Model file for the job. Use its own axes, mm. A direction names the side the tool comes from. Give positions to 0.01 mm unless a question says otherwise; leave off trailing zeros. Loops run counter-clockwise (first coordinate to the right, second up) from the corner with the lowest first, then second, coordinate; pieces in that order, holes last. Notation, with made-up numbers: M -26.5,29.5 L 7.5,29.5 A33 cw 7.5,61.5 Z; hole C 53.5,32 d2. An arc over 180 degrees is marked long. Answer in a Markdown table with one row per item.
```python
from build123d import *

# Parameters (mm, degrees)
EXTRUDE1_DEPTH      = 5.08
EXTRUDE1_DEPTH_BACK = 5.08
SKETCH3_R           = 9.525
SKETCH4_R           = 2.5796875
CUT_EXTRUDE1_DEPTH  = 37.55526843
FILLET1_R           = 2.54
FILLET2_R           = 2.54
CHAMFER1_SIZE       = 0.127
FILLET3_R           = 0.254
CHAMFER2_SIZE       = 0.127


with BuildPart() as part:
    # Sketch3 → Extrude1 (new, two sides: drawn at the far end of the back side and taken through both)
    with BuildSketch(Plane.XY.offset(-EXTRUDE1_DEPTH_BACK)):
        with BuildLine():
            Line((14.2875, 0), (14.2875, -7.9375))
            Line((14.2875, -7.9375), (28.575, -7.9375))
            Line((28.575, -7.9375), (28.575, -14.2875))
            Line((28.575, -14.2875), (-28.575, -14.2875))
            Line((-28.575, -14.2875), (-28.575, -7.9375))
            Line((-28.575, -7.9375), (-14.2875, -7.9375))
            Line((-14.2875, -7.9375), (-14.2875, 0))
            ThreePointArc((-14.2875, 0), (0, 14.2875), (14.2875, 0))
        make_face()
        Circle(SKETCH3_R, mode=Mode.SUBTRACT)
    extrude(amount=EXTRUDE1_DEPTH + EXTRUDE1_DEPTH_BACK)

    # Sketch4 → Cut-Extrude1 (cut, through all)
    with BuildSketch(Plane(origin=(0, -7.9375, 0), x_dir=(1, 0, 0), z_dir=(0, 1, 0))):
        with Locations(Location((-22.225, 0, 0), (0, 0, 270))):
            Circle(SKETCH4_R)
        with Locations(Location((22.225, 0, 0), (0, 0, 270))):
            Circle(SKETCH4_R)
        Polygon((-28.575, 5.08), (-28.575, 2.54), (-26.035, 5.08), align=None)
        Polygon((26.035, 5.08), (28.575, 5.08), (28.575, 2.54), align=None)
        Polygon((28.575, -5.08), (28.575, -2.54), (26.035, -5.08), align=None)
        Polygon((-26.035, -5.08), (-28.575, -5.08), (-28.575, -2.54), align=None)
    extrude(amount=-CUT_EXTRUDE1_DEPTH, mode=Mode.SUBTRACT)

    # Fillet1
    fillet1_edges = [part.edges().sort_by_distance(p)[0] for p in [
        (0, 14.2875, -5.08),
        (14.2875, -3.96875, -5.08),
        (14.2875, -3.96875, 5.08),
        (-14.2875, -3.96875, -5.08),
        (0, 14.2875, 5.08),
        (-14.2875, -3.96875, 5.08),
    ]]
    fillet(fillet1_edges, radius=FILLET1_R)

    # Fillet2
    # the kernel refuses this fillet: 2.54 mm, written as the material it adds along each edge
    with BuildSketch(Plane(origin=(-14.2875, -7.9375, -2.54), x_dir=(0, 1, 0), z_dir=(0, 0, 1)), Plane(origin=(14.2875, -7.9375, 2.54), x_dir=(0, 1, 0), z_dir=(0, 0, -1))) as fillet2_piece_1:
        with BuildLine():
            CenterArc((FILLET2_R, FILLET2_R), FILLET2_R, 180, 90)
            Line((0, FILLET2_R), (0, 0))
            Line((0, 0), (FILLET2_R, 0))
        make_face()
    extrude(amount=5.08)
    with BuildSketch(Plane(origin=(11.7475, -7.9375, -2.54), x_dir=(-0.5976672776328281, 0, 0.8017442392976479), z_dir=(0.8017442392976479, 0, 0.5976672776328281))) as fillet2_piece_2_section:
        with BuildLine():
            CenterArc((2.54 + FILLET2_R, -FILLET2_R), FILLET2_R, 90, 90)
            Line((2.54 + FILLET2_R, 0), (2.54, 0))
            Line((2.54, 0), (2.54, -FILLET2_R))
        make_face()
    fillet2_piece_2 = revolve(axis=Axis((11.7475, -7.9375, -2.54), (0, -1, 0)), revolution_arc=233.296989237, mode=Mode.PRIVATE)
    fillet2_piece_2 = split(fillet2_piece_2, bisect_by=Plane(origin=(13.652344814, -7.145963779, -5.08), z_dir=(0, 0, 1)), keep=Keep.TOP, mode=Mode.PRIVATE)
    add(fillet2_piece_2)
    with BuildSketch(Plane(origin=(-11.7475, -7.9375, -2.54), x_dir=(0.5976672776328252, 0, 0.8017442392976498), z_dir=(-0.8017442392976498, 0, 0.5976672776328252))) as fillet2_piece_3_section:
        with BuildLine():
            CenterArc((2.54 + FILLET2_R, FILLET2_R), FILLET2_R, 180, 90)
            Line((2.54, FILLET2_R), (2.54, 0))
            Line((2.54, 0), (2.54 + FILLET2_R, 0))
        make_face()
    fillet2_piece_3 = revolve(axis=Axis((-11.7475, -7.9375, -2.54), (0, 1, 0)), revolution_arc=233.296989237, mode=Mode.PRIVATE)
    fillet2_piece_3 = split(fillet2_piece_3, bisect_by=Plane(origin=(-13.652344909, -7.145964282, -5.08), z_dir=(0, 0, 1)), keep=Keep.TOP, mode=Mode.PRIVATE)
    add(fillet2_piece_3)
    with BuildSketch(Plane(origin=(11.7475, -7.9375, 2.54), x_dir=(1, 0, 0), z_dir=(0, 0, -1))) as fillet2_piece_4_section:
        with BuildLine():
            CenterArc((2.54 + FILLET2_R, -FILLET2_R), FILLET2_R, 90, 90)
            Line((2.54 + FILLET2_R, 0), (2.54, 0))
            Line((2.54, 0), (2.54, -FILLET2_R))
        make_face()
    fillet2_piece_4 = revolve(axis=Axis((11.7475, -7.9375, 2.54), (0, -1, 0)), revolution_arc=233.296989237, mode=Mode.PRIVATE)
    fillet2_piece_4 = split(fillet2_piece_4, bisect_by=Plane(origin=(13.65234485, -7.145963968, 5.08), z_dir=(0, 0, -1)), keep=Keep.TOP, mode=Mode.PRIVATE)
    add(fillet2_piece_4)
    with BuildSketch(Plane(origin=(-11.7475, -7.9375, 2.54), x_dir=(-1, 0, 0), z_dir=(0, 0, -1))) as fillet2_piece_5_section:
        with BuildLine():
            CenterArc((2.54 + FILLET2_R, FILLET2_R), FILLET2_R, 180, 90)
            Line((2.54, FILLET2_R), (2.54, 0))
            Line((2.54, 0), (2.54 + FILLET2_R, 0))
        make_face()
    fillet2_piece_5 = revolve(axis=Axis((-11.7475, -7.9375, 2.54), (0, 1, 0)), revolution_arc=233.296989237, mode=Mode.PRIVATE)
    fillet2_piece_5 = split(fillet2_piece_5, bisect_by=Plane(origin=(-14.845729139, -7.512557487, 5.08), z_dir=(0, 0, -1)), keep=Keep.TOP, mode=Mode.PRIVATE)
    add(fillet2_piece_5)

    # Chamfer1
    chamfer1_edges = [part.edges().sort_by_distance(p)[0] for p in [
        (-9.525, 0, 5.08),
        (-9.525, 0, -5.08),
    ]]
    chamfer(chamfer1_edges, length=CHAMFER1_SIZE)

    # Sketch5 → Revolve1 (revolve)
    with BuildSketch(Plane(origin=(0, 0, 0), x_dir=(0, 0, -1), z_dir=(1, 0, 0))):
        Polygon((-4.826, 9.525), (-4.826, 8.334375), (-5.08, 8.334375), (-5.08, 5.953125), (-4.826, 5.953125), (-4.826, 4.7625), (4.826, 4.7625), (4.826, 5.953125), (5.08, 5.953125), (5.08, 8.334375), (4.826, 8.334375), (4.826, 9.525), align=None)
    revolve(axis=Axis((0, 0, 0), (0, 0, 1)))

    # Fillet3
    fillet3_edges = [part.edges().sort_by_distance(p)[0] for p in [
        (0, -4.7625, -4.826),
        (0, -4.7625, 4.826),
    ]]
    fillet(fillet3_edges, radius=FILLET3_R)

    # Chamfer2
    chamfer2_edges = [part.edges().sort_by_distance(p)[0] for p in [
        (0, -8.334375, -5.08),
        (0, -5.953125, -5.08),
        (0, -5.953125, 5.08),
        (0, -8.334375, 5.08),
    ]]
    chamfer(chamfer2_edges, length=CHAMFER2_SIZE)


solid = part.part
```
Q1. Mould opens along Z. For faces 1 (the face through (13.56, -2.74, -4.32)), 2 (the face through (6, 6, 4.826)), 3 (the face through (-28.575, -11, 0)), 4 (the face through (24.783, -11.068, -0.336)) say: released by +Z, released by -Z, zero draft, split by the parting line, or undercut.
Reported:
| item | result |
|---|---|
| face 1 | released by -Z |
| face 2 | released by +Z |
| face 3 | zero draft |
| face 4 | undercut |
Q2. Saw through at A-A (z = 0). Give the cut face in (x, y) (1 decimal), and give its area (3 significant figures).
Reported:
| item | result |
|---|---|
| outline | M -28.6,-14.3 L -24.8,-14.3 L -24.8,-7.9 L -28.6,-7.9 Z; M -19.6,-14.3 L 19.6,-14.3 L 19.6,-7.9 L 16.8,-7.9 A2.5 cw 14.3,-5.4 L 14.3,0 A14.3 ccw -14.3,0 L -14.3,-5.4 A2.5 cw -16.8,-7.9 L -19.6,-7.9 Z; M 24.8,-14.3 L 28.6,-14.3 L 28.6,-7.9 L 24.8,-7.9 Z; hole C 0,0 d9.5 |
| area | 776 mm² |
Q3. Drop flat-ended pins along their axis: pin 1 (4.5 mm diameter, centred on x = -22.225, z = 0, fed in from -Y); pin 2 (15.5 mm diameter, centred on x = 0, y = 0, fed in from -Z); pin 3 (1.5 mm diameter, centred on y = -2.5, z = 1, fed in from +X); pin 4 (1 mm diameter, centred on x = -21.5, z = -3.5, fed in from +Y). Give the stop position or say it passes through.
Reported:
| item | result |
|---|---|
| pin 1 | through |
| pin 2 | z = -5.08 |
| pin 3 | x = 14.29 |
| pin 4 | y = -7.94 |
Q4. Probe probe 1 along X at (y, z) = (-11, 0) (3 decimals); probe 2 along Z at (x, y) = (22, -10); probe 3 along Y at (x, z) = (22, -3.5). List the from-to ranges inside material, lowest first.
Reported:
| item | result |
|---|---|
| probe 1 | -28.575 to -24.805, -19.645 to 19.645, 24.805 to 28.575 |
| probe 2 | -5.08 to -2.57, 2.57 to 5.08 |
| probe 3 | -14.29 to -7.94 |
Q5. 3-axis set-ups, long thin cutter, end or side, ignore diameter. For faces 5 (the face through (13.56, -2.74, 4.32)), 6 (the face through (14.288, -3, 0)), 7 (the face through (5, -2, -4.826)), 8 (the face through (-13.56, -2.66, 4.32)), 9 (the face through (5, 2, 4.826)): which of +Z, -Z, +X, -X, +Y, -Y reach the whole face in a straight line?
Reported:
| item | result |
|---|---|
| face 5 | +Z, +X, +Y |
| face 6 | +Z, -Z, +X, +Y |
| face 7 | -Z |
| face 8 | +Z, -X, +Y |
| face 9 | +Z |
